Autodesk Inventor part; units mm, degrees
ref_plane "Arbeitsebene1" through (-51, 0, 12) normal (0, 0, -1) x (-1, 0, 0)
ref_plane "YZ Plane" through (0, 0, 0) normal (1, 0, 0) x (0, 1, 0)
ref_plane "XZ Plane" through (0, 0, 0) normal (0, 1, 0) x (-1, 0, 0)
sketch "Skizze1" plane through (0, 0, 0) normal (0, 1, 0) x (-1, 0, 0)
  line L0 (-54, 0) -> (54, 0)
  line L1 (54, 0) -> (54, 24)
  line L2 (54, 24) -> (21, 24)
  line L3 (21, 24) -> (21, 47)
  line L4 (21, 47) -> (-21, 47)
  line L5 (-21, 47) -> (-21, 24)
  line L6 (-21, 24) -> (-54, 24)
  line L7 (-54, 24) -> (-54, 0)
  point P0 (0, 0)
  point P1 (0, 0)
  dimension "d0" = 108
  dimension "d1" = 24
  dimension "d2" = 33
  dimension "d3" = 23
  dimension "d4" = 42
extrude "Extrusion1" add sketch "Skizze1" along normal blind 5
sketch "Skizze2" plane through (54, 0, 24) normal (1, 0, 0) x (0, 0, -1)
  line L0 (0, 0) -> (24, 0)
  line L1 (24, 0) -> (24, 5)
  line L2 (0, 5) -> (24, 5)
  line L3 (0, 0) -> (0, 5)
  line L4 (2, 0) -> (22, 0)
  line L5 (22, 0) -> (22, 5)
  line L6 (22, 5) -> (2, 5)
  line L7 (2, 5) -> (2, 0)
  dimension "d7" = 2
  dimension "d8" = 2
extrude "Extrusion2" cut sketch "Skizze2" against normal blind 3 contours L7 L2 L5 L0
sketch "Skizze3" plane through (-54, 0, 0) normal (-1, 0, 0) x (0, 0, 1)
  line L0 (0, 0) -> (24, 0)
  line L1 (24, 0) -> (24, 5)
  line L2 (0, 5) -> (24, 5)
  line L3 (0, 0) -> (0, 5)
  line L4 (2, 0) -> (22, 0)
  line L5 (22, 0) -> (22, 5)
  line L6 (22, 5) -> (2, 5)
  line L7 (2, 5) -> (2, 0)
  dimension "d11" = 2
  dimension "d12" = 2
extrude "Extrusion3" cut sketch "Skizze3" against normal blind 3 contours L7 L2 L5 L0
fillet "Rundung1" radius 1 8 edges at (-54, 2.5, 0) (-54, 2.5, 2) (-54, 2.5, 22) (-54, 2.5, 24) (54, 2.5, 24) (54, 2.5, 22) (54, 2.5, 2) (54, 2.5, 0)
fillet "Rundung2" radius 5 4 edges at (21, 2.5, 24) (21, 2.5, 47) (-21, 2.5, 47) (-21, 2.5, 24)
sketch "Skizze4" plane through (53, 0, 0) normal (0, 0, -1) x (-1, 0, 0)
  line L0 (58.5, -0.5) -> (47.5, -0.5)
  line L1 (47.5, -0.5) -> (47.5, 0.5)
  line L2 (47.5, 0.5) -> (58.5, 0.5)
  line L3 (58.5, 0.5) -> (58.5, -0.5)
  line L4 (58.5, -0.5) -> (47.5, 0.5) construction
  line L5 (47.5, -0.5) -> (58.5, 0.5) construction
  point P0 (53, 0)
  dimension "d17" = 11
  dimension "d18" = 1
extrude "Extrusion4" cut sketch "Skizze4" against normal through all
sketch "Skizze6" plane through (0, 5, 0) normal (0, 1, 0) x (1, 0, 0)
  line L0 (53, 0) -> (-53, 0)
  point P0 (0, 0)
  point P1 (-26, -12)
  point P2 (26, -12)
  dimension "d31" = 12
  dimension "d32" = 26
  dimension "d33" = 26
hole "Bohrung2" at (-26, 5, 12) at (26, 5, 12) direction (0, -1, 0) diameter 4.2 end through all countersink diameter 8.4 countersink angle 90
sketch "Skizze7" plane through (51, 0, 24) normal (1, 0, 0) x (0, 0, -1)
  line L0 (22, 5) -> (22, 0)
  line L1 (2, 5) -> (22, 5)
  point P0 (24, 0)
  point P1 (12, 2.5)
  dimension "d41" = 2.5
  dimension "d42" = 10
hole "Bohrung3" at (51, 2.5, 12) direction (-1, 0, 0) diameter 2.459 depth 6 tip angle 118
sketch "Skizze8" plane through (-51, 0, 0) normal (-1, 0, 0) x (0, 0, 1)
  line L0 (2, 5) -> (22, 5)
  line L1 (2, 0) -> (2, 5)
  point P0 (0, 0)
  point P1 (12, 2.5)
  dimension "d50" = 2.5
  dimension "d51" = 10
hole "Bohrung4" at (-51, 2.5, 12) direction (1, 0, 0) diameter 2.459 depth 6 tip angle 118
ref_plane "Arbeitsebene1" through (-51, 0, 12) normal (0, 0, -1) x (-1, 0, 0)
fillet "Rundung3" radius 2 2 edges at (51, 2.5, 2) (51, 2.5, 22)
fillet "Rundung4" radius 2 2 edges at (-51, 2.5, 22) (-51, 2.5, 2)
properties part number "Grundplatte"
The model under review builds one solid part; all positions refer to its coordinate system, in mm. A direction names the side the tool comes from. Round coordinates to 2 decimals unless told otherwise and drop trailing zeros. Order: outer loops, then holes, each group sorted by start corner. A loop starts at its lowest first (then second) coordinate and runs counter-clockwise, first axis right, second up.
Item 1: For pin 1 (12 mm diameter, centred on x = -1, z = 29.5, fed in from -Y); pin 2 (3.5 mm diameter, centred on x = 26, z = 12, fed in from -Y); pin 3 (2.5 mm diameter, centred on y = 1.5, z = 11.5, fed in from +X); pin 4 (1 mm diameter, centred on y = 1.5, z = 10, fed in from -X), all flat-tipped, find the tip position at first contact; note any pin that passes through.
Working result:
pin 1: stops at y = 0
pin 2: passes through
pin 3: stops at x = 51
pin 4: stops at x = -51
Item 2: Machinability: for faces 4 (the flat face through (-40, 2, 24)), 5 (the flat face through (0, 0.5, 23)), 6 (the cylindrical face through (-51.6, 2.46, 2.57)), which of the approach directions +Z, -Z, +X, -X, +Y, -Y give a long, thin tool a straight path to every point of the face, cutting with its end or side? Answer none if there is none.
Working result:
face 4: +Z, -X, +Y, -Y
face 5: +Z, -Z, -Y
face 6: -X, +Y, -Y
Item 3: Add section B-B, the plane x = -4. State the section outline as (y, z) points.
Working result:
outline: (0.5, 0) - (5, 0) - (5, 47) - (0.5, 47) - close
Item 4: To check wall thickness, follow probe 1 along Z at (x, y) = (49.05, 2.5); probe 2 along Z at (x, y) = (26, 0.85); probe 3 along X at (y, z) = (4.55, 10.5). State the ranges of each line that lie inside material, in increasing order.
Working result:
probe 1: z = 0 to 10.77, 13.23 to 24
probe 2: z = 0 to 9.9, 14.1 to 24
probe 3: x = -51 to -29.44, -22.56 to 22.56, 29.44 to 51
Item 5: Add section A-A, the plane x = 36. State the section outline as (y, z) points.
Working result:
outline: (0, 0) - (5, 0) - (5, 24) - (0, 24) - close
Item 6: Draft analysis for pull direction Y (two halves, no side actions). For faces 1 (the cylindrical face through (23, 3, 25)), 2 (the flat face through (1, 5, 19)), 3 (the cylindrical face through (47.958, 2.131, 10.827)), state which applies: released by +Y, released by -Y, zero draft, split by the parting line, or undercut.
Working result:
face 1: zero draft
face 2: released by +Y
face 3: undercut
